from build123d import *

# Parameters (mm, degrees)
F0_W     = 56.778665632
F0_H     = 40.8155359328
F1_DEPTH = 10
F3_D     = 4
F3_DEPTH = 5
F3_TIP   = 1.2017212381
F4_R     = 8.0897194279
F5_DEPTH = 25.4


with BuildPart() as f1:
    # F0 (on Top) → F1 (new body)
    with BuildSketch(Plane.XY):
        with Locations((28.389332816, 20.4077679664)):
            Rectangle(F0_W, F0_H)
    extrude(amount=F1_DEPTH)

    # F3
    with Locations(Plane.XY.offset(10)):
        with Locations((25.281002745, 19.7033435106)):
            Hole(F3_D / 2, depth=F3_DEPTH)
            with Locations((0, 0, -(F3_DEPTH + F3_TIP / 2))):  # 118° drill point
                Cone(0, F3_D / 2, F3_TIP, mode=Mode.SUBTRACT)

    # F4 (on face) → F5 (join)
    with BuildSketch(Plane.XY.offset(10)):
        with Locations((33.39304775, 27.8067756444)):
            Circle(F4_R)
    extrude(amount=F5_DEPTH)


solid = f1.part
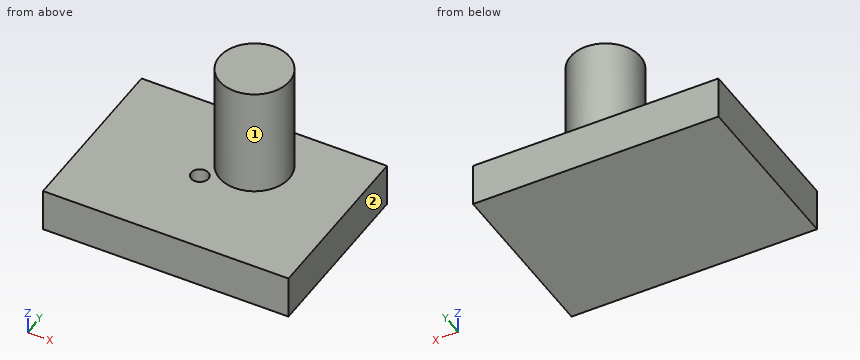
Can you work these out from the model? Positions are in its coordinate system, mm. Face numbers are marked on the shaded views. A direction names the side the tool comes from. Give positions to 0.01 mm unless a question says otherwise; leave off trailing zeros. Loops run counter-clockwise (first coordinate to the right, second up) from the corner with the lowest first, then second, coordinate; pieces in that order, holes last. Notation, with made-up numbers: (-0.5, -29.5) -> (19.5, -29.5) arc R16 ccw to (19.5, -0.5) -> close; hole circle Ø7 at (-14.75, 68.5). An arc over 180 degrees is marked (long way). Use one line per item in the form item = value.
1) Will these pins go through, and if not, where does the flat tip stop? pin 1 (1.5 mm diameter, centred on x = 35, z = 23.5, fed in from +Y); pin 2 (3.5 mm diameter, centred on x = 25.28, y = 19.7, fed in from +Z); pin 3 (8 mm diameter, centred on x = 45, y = 19.5, fed in from +Z).
Answers:
pin_1 = 35.85
pin_2 = 4.85
pin_3 = 10
2) If we section it at C-C (z = 23): Please give me the cut outline in (x, y), plus the area to 3 significant figures.
Answers:
outline = circle Ø16.18 at (33.39, 27.81)
area = 206 mm²
3) If we section it at D-D (y = 12.5): Please give me the cut outline in (x, z).
Answers:
outline = (0, 0) -> (56.78, 0) -> (56.78, 10) -> (0, 10) -> close
4) If we section it at A-A (x = 38): Please give me the cut outline in (y, z), plus the area to 3 significant figures.
Answers:
outline = (0, 0) -> (40.82, 0) -> (40.82, 10) -> (34.46, 10) -> (34.46, 35.4) -> (21.16, 35.4) -> (21.16, 10) -> (0, 10) -> close
area = 746 mm²
5) For the marked faces 1 and 2, which set-ups out of +Z, -Z, +X, -X, +Y, -Y let a thin tool reach every point of the face, with its end or its side?
Answers:
face_1 = +Z
face_2 = +Z, -Z, +X, +Y, -Y
6) I need wall thicknesses on line 1 along Z through (x, y) = (54, 32.5); line 2 along Y through (x, z) = (29, 25.5); line 3 along X through (y, z) = (32, 31). Which ranges of each line are inside material? Lowest first, please.
Answers:
line_1 = 0 to 10
line_2 = 21.01 to 34.6
line_3 = 26.47 to 40.31
7) If we section it at B-B (y = 25.5): Please give me the cut outline in (x, z), plus the area to 3 significant figures.
Answers:
outline = (0, 0) -> (56.78, 0) -> (56.78, 10) -> (41.15, 10) -> (41.15, 35.4) -> (25.64, 35.4) -> (25.64, 10) -> (0, 10) -> close
area = 962 mm²
